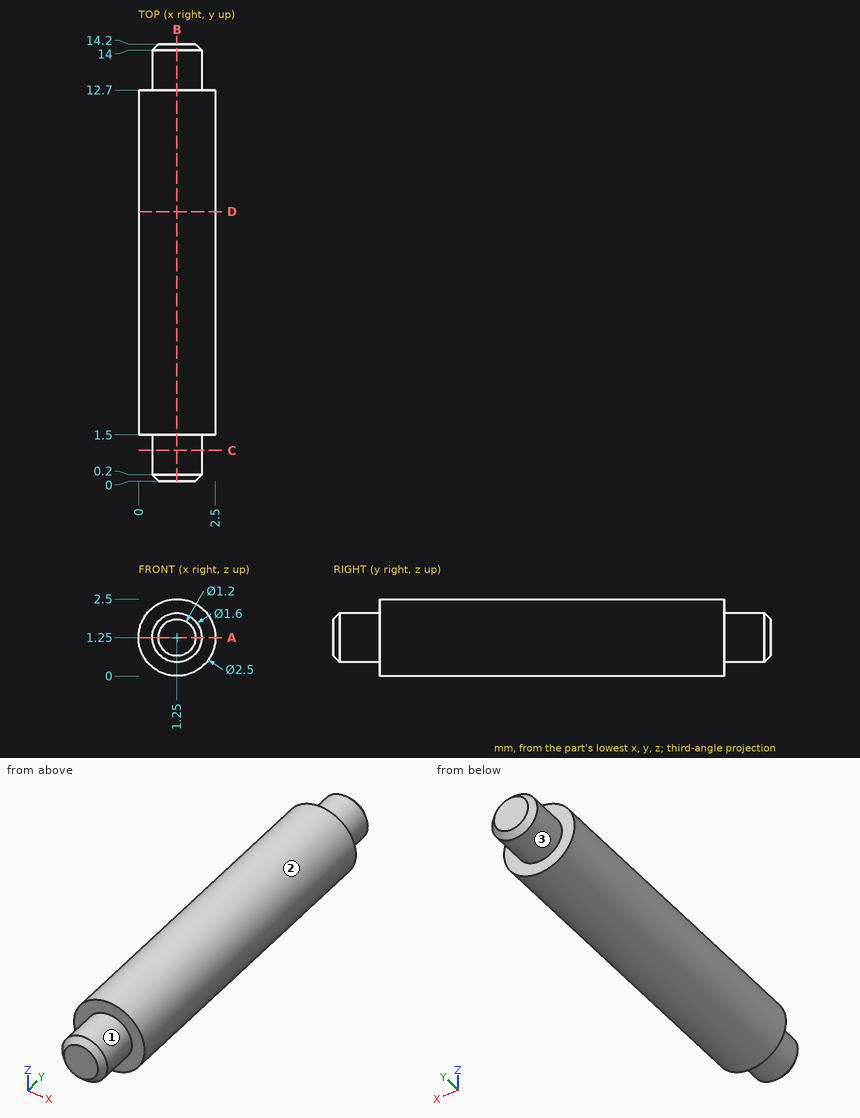
Can you work these out from the drawing? Everything is in mm from the part's minimum corner. A direction names the side the tool comes from. Coordinates: 2 decimals unless noted, no trailing zeros. Loops run counter-clockwise (first coordinate to the right, second up) from the corner with the lowest first, then second, coordinate; pieces in that order, holes last.
1) Imagine slicing it at A-A on z = 1.25. List the corners of the cut face in (x, y) for me, plus the area to 3 significant figures.
2) For pin 1 (1 mm diameter, centred on x = 0.5, y = 4.5, fed in from -Z), with a flat end and sliding along its axis, tell me the tip position at first contact or that it passes through.
3) Which directions (+Z, -Z, +X, -X, +Y, -Y) give clear straight access to the entire face, cutting with the end or side of a thin tool? Please do the marked faces 1, 2 and 3.
4) Imagine slicing it at C-C on y = 1. List the corners of the cut face in (x, z) for me, plus the area to 3 significant figures.
5) I need wall thicknesses on probe 1 along Y at (x, z) = (0.2, 1.7); probe 2 along Z at (x, y) = (0.2, 7.5); probe 3 along Z at (x, y) = (1.9, 12.5). Which ranges of each line are inside material? Lowest first, please.
6) Imagine slicing it at D-D on y = 8.75. List the corners of the cut face in (x, z) for me, plus the area to 3 significant figures.
7) Imagine slicing it at B-B on x = 1.25. List the corners of the cut face in (y, z) for me.
Completed:
1. outline: (0, 1.5) - (0.45, 1.5) - (0.45, 0.2) - (0.65, 0) - (1.85, 0) - (2.05, 0.2) - (2.05, 1.5) - (2.5, 1.5) - (2.5, 12.7) - (2.05, 12.7) - (2.05, 14) - (1.85, 14.2) - (0.65, 14.2) - (0.45, 14) - (0.45, 12.7) - (0, 12.7) - close
1. area: 32.7 mm2
2. pin 1: stops at z = 0.03
3. face 1: -Y
3. face 2: +Y, -Y
3. face 3: +Y
4. outline: circle Ø1.6 at (1.25, 1.25)
4. area: 2.01 mm2
5. probe 1: y = 1.5 to 12.7
5. probe 2: z = 0.57 to 1.93
5. probe 3: z = 0.18 to 2.32
6. outline: circle Ø2.5 at (1.25, 1.25)
6. area: 4.91 mm2
7. outline: (0, 0.65) - (0.2, 0.45) - (1.5, 0.45) - (1.5, 0) - (12.7, 0) - (12.7, 0.45) - (14, 0.45) - (14.2, 0.65) - (14.2, 1.85) - (14, 2.05) - (12.7, 2.05) - (12.7, 2.5) - (1.5, 2.5) - (1.5, 2.05) - (0.2, 2.05) - (0, 1.85) - close
